For this review, use the dimensioned drawing (mm, ordinates from the lowest corner) and the shaded views. Give positions to 0.01 mm unless a question says otherwise; leave off trailing zeros. Loops run counter-clockwise (first coordinate to the right, second up) from the corner with the lowest first, then second, coordinate; pieces in that order, holes last. Notation, with made-up numbers: (76, 59.25) - (97, 59.25) arc R18 cw to (97, 87.25) - close; hole circle Ø11 at (14.25, -34). An arc over 180 degrees is marked (long way). Write each question's results on one line, items separated by ' | '.
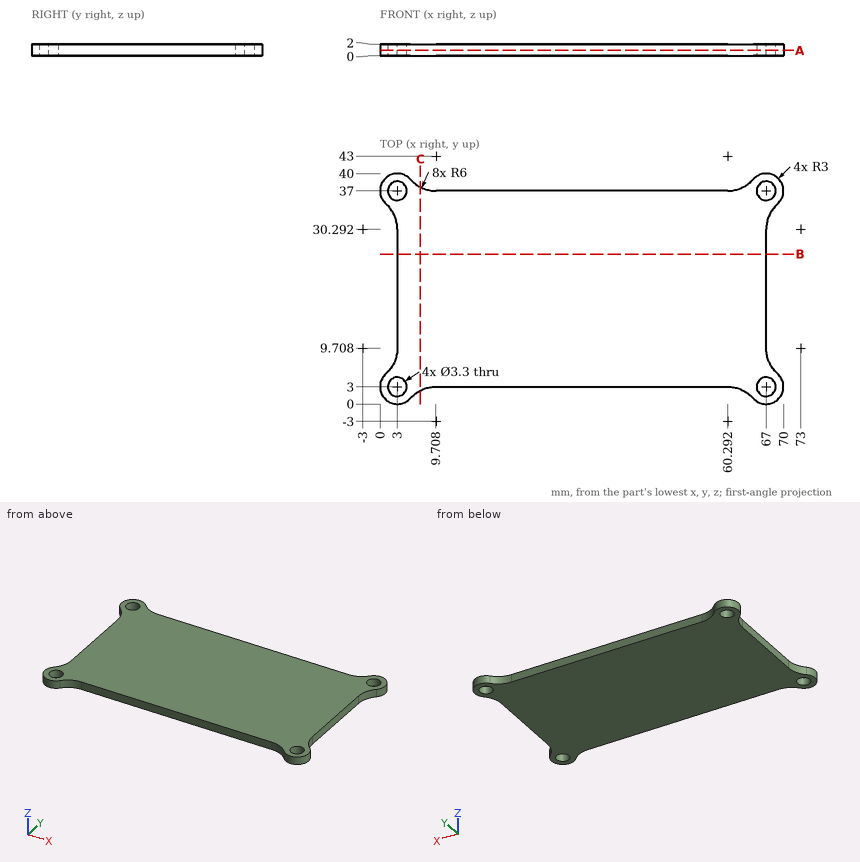
Item 1: We need section C-C on x = 7. Give the boundary of the cut face in (y, z), then the cut area to 3 significant figures.
Output values:
outline: (2.35, 0) - (37.65, 0) - (37.65, 2) - (2.35, 2) - close | area: 70.6 mm²
Item 2: We need section B-B on y = 26. Give the boundary of the cut face in (x, z), then the cut area to 3 significant figures.
Output values:
outline: (3, 0) - (67, 0) - (67, 2) - (3, 2) - close | area: 128 mm²
Item 3: Wall thickness on probe 1 along X at (y, z) = (2.5, 1); probe 2 along X at (y, z) = (4.5, 0.5); probe 3 along Y at (x, z) = (4, 1.25): over which ranges is each line inside the solid? List them lowest first.
Output values:
probe 1: x = 0.04 to 1.43, 4.57 to 7.31, 62.69 to 65.43, 68.57 to 69.96 | probe 2: x = 0.4 to 2.31, 3.69 to 66.31, 67.69 to 69.6 | probe 3: y = 0.17 to 1.69, 4.31 to 35.69, 38.31 to 39.83
Item 4: Clearance check with flat-ended pins moving along their axes: P1, Ø5.5, axis at x = 3, y = 3, coming from the +Z side; P2, Ø1, axis at x = 43.5, z = 1.5, coming from the -Y side; P3, Ø0.6, axis at y = 16.5, z = 1, coming from the +X side. State where each tip first meets the part, or that it passes through.
Output values:
P1: stops at z = 2 | P2: stops at y = 3 | P3: stops at x = 67
Item 5: We need section A-A on z = 0.9. Give the boundary of the cut face in (x, y), then the cut area to 3 significant figures.
Output values:
outline: (1, 5.24) arc R3 ccw (long way) to (5.24, 1) arc R6 cw to (9.71, 3) - (60.29, 3) arc R6 cw to (64.76, 1) arc R3 ccw (long way) to (69, 5.24) arc R6 cw to (67, 9.71) - (67, 30.29) arc R6 cw to (69, 34.76) arc R3 ccw (long way) to (64.76, 39) arc R6 cw to (60.29, 37) - (9.71, 37) arc R6 cw to (5.24, 39) arc R3 ccw (long way) to (1, 34.76) arc R6 cw to (3, 30.29) - (3, 9.71) arc R6 cw to start; hole circle Ø3.3 at (3, 3); hole circle Ø3.3 at (3, 37); hole circle Ø3.3 at (67, 3); hole circle Ø3.3 at (67, 37) | area: 2,240 mm²
